Part model, mm, in its own coordinate system. Face numbers are marked on the shaded views. A direction names the side the tool comes from. Round coordinates to 2 decimals unless told otherwise and drop trailing zeros. Order: outer loops, then holes, each group sorted by start corner. A loop starts at its lowest first (then second) coordinate and runs counter-clockwise, first axis right, second up. Notation, with made-up numbers: (21, -37) -> (78, -37) arc R33 ccw to (78, -9) -> close; hole circle Ø10 at (78.25, 25). An arc over 180 degrees is marked (long way). Use CSV: the item, a comma, the result in double quotes.
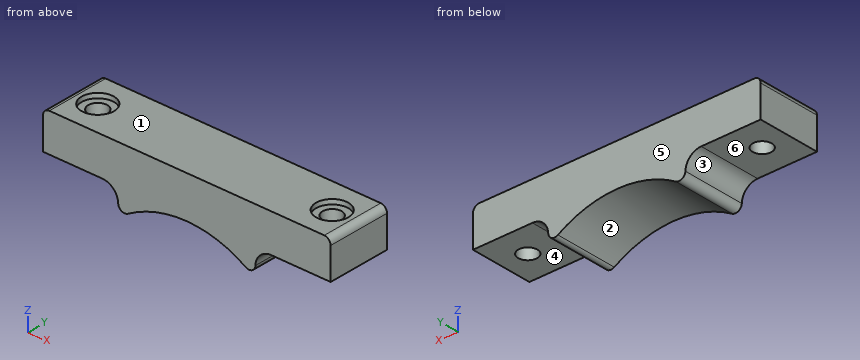
```python
from build123d import *

# Parameters (mm, degrees)
BOSS_EXTRUDE1_DEPTH = 20
FILLET1_R           = 2
HOLE1_D             = 6
HOLE1_DEPTH         = 20.26
HOLE1_CBORE_D       = 10.2
HOLE1_CBORE_DEPTH   = 1.5
HOLE1_TIP           = 1.802581857
FILLET2_R           = 2


with BuildPart() as part:
    # Sketch1 → Boss-Extrude1 (new body)
    with BuildSketch(Plane(origin=(0, 0, 0), x_dir=(1, 0, 0), z_dir=(0, 1, 0))):
        with BuildLine():
            Line((45.4, 0), (-45.4, 0))
            Line((-45.4, 0), (-45.4, 12))
            Line((-45.4, 12), (-26.65, 12))
            ThreePointArc((-26.65, 12), (-23.114466094, 13.464466094), (-21.65, 17))
            Line((-21.65, 17), (-21.65, 20.565901472))
            ThreePointArc((-21.65, 20.565901472), (0, 13.2), (21.65, 20.565901472))
            Line((21.65, 20.565901472), (21.65, 17))
            ThreePointArc((21.65, 17), (23.114466094, 13.464466094), (26.65, 12))
            Line((26.65, 12), (45.4, 12))
            Line((45.4, 12), (45.4, 0))
        make_face()
    extrude(amount=BOSS_EXTRUDE1_DEPTH)

    # Fillet1
    fillet1_edges = [part.edges().sort_by_distance(p)[0] for p in [
        (21.65, 10, -20.565901472),
        (-21.65, 10, -20.565901472),
    ]]
    fillet(fillet1_edges, radius=FILLET1_R)

    # Hole1
    with Locations(Plane.XY):
        with Locations((-37, 10), (37, 10)):
            CounterBoreHole(HOLE1_D / 2, HOLE1_CBORE_D / 2, HOLE1_CBORE_DEPTH, depth=HOLE1_DEPTH)
            with Locations((0, 0, -(HOLE1_DEPTH + HOLE1_TIP / 2))):  # 118° drill point
                Cone(0, HOLE1_D / 2, HOLE1_TIP, mode=Mode.SUBTRACT)

    # Fillet2
    fillet2_edges = [part.edges().sort_by_distance(p)[0] for p in [
        (45.4, 10, 0),
        (-45.4, 10, 0),
    ]]
    fillet(fillet2_edges, radius=FILLET2_R)


solid = part.part
```
(1) Drop flat-ended pins along their axis: P1, Ø5, axis at x = -37.5, y = 8.5, coming from the +Z side; P2, Ø8, axis at x = 37, y = 10, coming from the -Z side; P3, Ø4, axis at x = -2, y = 10.5, coming from the -Z side. Give the stop position or say it passes through.
Reply:
P1,"z = -1.5"
P2,"z = -12"
P3,"z = -13.43"
(2) Cut at B-B, the plane z = -8.25. Give the cut face in (x, y).
Reply:
outline,"(-45.4, 0) -> (45.4, 0) -> (45.4, 20) -> (-45.4, 20) -> close; hole circle Ø6 at (-37, 10); hole circle Ø6 at (37, 10)"
(3) Cut at D-D, the plane x = 11. Give the cut face in (y, z).
Reply:
outline,"(0, -14.95) -> (20, -14.95) -> (20, 0) -> (0, 0) -> close"
(4) Pull direction X, two halves, no side cores. Call the marked faces 1, 2 and 3: released by +X, released by -X, zero draft, split by the parting line, or undercut.
Reply:
face 1,"zero draft"
face 2,"undercut"
face 3,"released by -X"
(5) Cut at A-A, the plane x = -37. Give the cut face in (y, z), then the cut area to 3 significant figures.
Reply:
outline,"(0, -12) -> (7, -12) -> (7, -1.5) -> (4.9, -1.5) -> (4.9, 0) -> (0, 0) -> close; (13, -12) -> (20, -12) -> (20, 0) -> (15.1, 0) -> (15.1, -1.5) -> (13, -1.5) -> close"
area,"162 mm2"
(6) Cut at C-C, the plane y = 10. State how many separate pieces and enclosed holes the cut face has, then the cut area to 3 significant figures.
Reply:
separate pieces,"3"
enclosed holes,"0"
area,"1,090 mm2"
(7) Probe probe 1 along X at (y, z) = (12.5, -8); probe 2 along Z at (x, y) = (-33, 12); probe 3 along Y at (x, z) = (37, -8.75). List the from-to ranges inside material, lowest first. Write a range as [from, to].
Reply:
probe 1,"[-45.4, -38.66], [-35.34, 35.34], [38.66, 45.4]"
probe 2,"[-12, -1.5]"
probe 3,"[0, 7], [13, 20]"
(8) Which spindle directions (+Z, -Z, +X, -X, +Y, -Y) get a long thin tool onto all of the face, cutting with end or side? Do the marked faces 4, 5 and 6. Say none if no direction does.
Reply:
face 4,"-Z, +X, +Y, -Y"
face 5,"+Z, -Z, +X, -X, +Y"
face 6,"-Z, -X, +Y, -Y"
